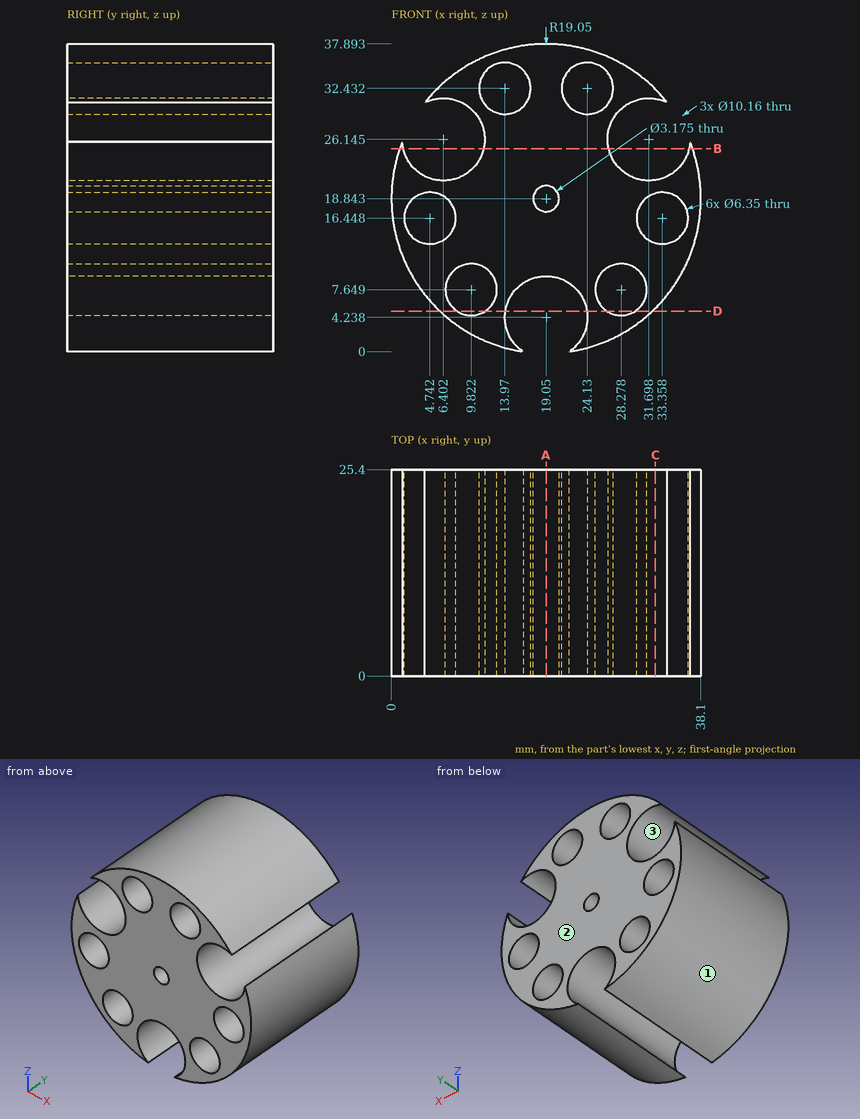
Can you work these out from the drawing? Everything is in mm from the part's minimum corner. Give positions to 0.01 mm unless a question says otherwise; leave off trailing zeros. Order: outer loops, then holes, each group sorted by start corner. A loop starts at its lowest first (then second) coordinate and runs counter-clockwise, first axis right, second up. Notation, with made-up numbers: M 78.5,-13 L 96.5,-13 A27 ccw 96.5,18 Z; hole C 21.25,41.25 d8. An arc over 180 degrees is marked long. Use a Markdown table: item, result. Add a question column.
Item 1: Suppose I cut it at A-A (x = 19.05). List the corners of the cut face in (y, z) for me (1 decimal).
Item 2: Suppose I cut it at D-D (z = 5). List the corners of the cut face in (x, y) for me, then the cut area to 3 significant figures.
Item 3: Suppose I cut it at B-B (z = 25). List the corners of the cut face in (x, y) for me, then the cut area to 3 significant figures.
Item 4: We'd pull the mould along X, two halves only. Please class the marked faces 1, 2 and 3: +X half, -X half, draft (parallel to the pull), parting line (faces both ways), or undercut.
Item 5: Will these pins go through, and if not, where does the flat tip stop? pin 1 (8 mm diameter, centred on x = 28, y = 5.5, fed in from +Z); pin 2 (3 mm diameter, centred on x = 21.5, y = 21, fed in from +Z); pin 3 (3 mm diameter, centred on x = 26.5, y = 12.5, fed in from +Z).
Item 6: If I drill on L1, parallel to Z at x = 26.5, y = 19.5 (1 decimal); L2, parallel to X at y = 17.75, z = 25.5; L3, parallel to X at y = 2.5, z = 17 (1 decimal), over which ranges is the centre line in solid material (lowest first)? Write a range as [from, to].
Item 7: Suppose I cut it at C-C (x = 32.5). List the corners of the cut face in (y, z) for me (1 decimal).
Answer sheet:
| question | item | result |
|---|---|---|
| 1 | outline | M 0,9.3 L 25.4,9.3 L 25.4,17.3 L 0,17.3 Z; M 0,20.4 L 25.4,20.4 L 25.4,37.9 L 0,37.9 Z |
| 2 | outline | M 5.96,0 L 8.07,0 L 8.07,25.4 L 5.96,25.4 Z; M 11.57,0 L 14.03,0 L 14.03,25.4 L 11.57,25.4 Z; M 24.07,0 L 26.53,0 L 26.53,25.4 L 24.07,25.4 Z; M 30.03,0 L 32.14,0 L 32.14,25.4 L 30.03,25.4 Z |
| 2 | area | 232 mm² |
| 3 | outline | M 1.02,0 L 1.45,0 L 1.45,25.4 L 1.02,25.4 Z; M 11.35,0 L 26.75,0 L 26.75,25.4 L 11.35,25.4 Z; M 36.65,0 L 37.08,0 L 37.08,25.4 L 36.65,25.4 Z |
| 3 | area | 413 mm² |
| 4 | face 1 | -X half |
| 4 | face 2 | draft |
| 4 | face 3 | undercut |
| 5 | pin 1 | stops at z = 37.24 |
| 5 | pin 2 | stops at z = 37.87 |
| 5 | pin 3 | stops at z = 36.94 |
| 6 | L1 | z = [1.3, 5], [10.3, 30.3], [34.5, 36.4] |
| 6 | L2 | x = [1.2, 1.36], [11.44, 26.66], [36.74, 36.9] |
| 6 | L3 | x = [0.1, 1.6], [7.9, 30.2], [36.5, 38] |
| 7 | outline | M 0,5.4 L 25.4,5.4 L 25.4,13.4 L 0,13.4 Z; M 0,19.5 L 25.4,19.5 L 25.4,21.1 L 0,21.1 Z; M 0,31.2 L 25.4,31.2 L 25.4,32.3 L 0,32.3 Z |
